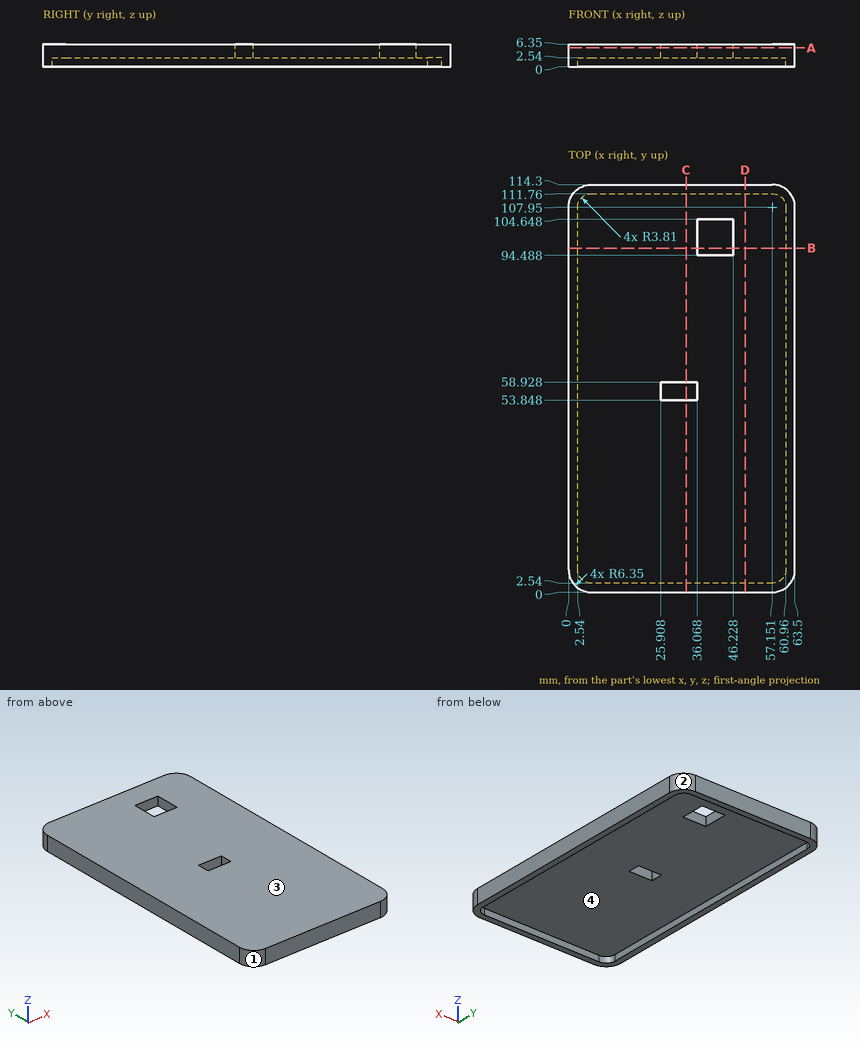
Print and shaded views of the part. All mm, measured from the part's lowest x, y and z. Coordinates: 2 decimals unless noted, no trailing zeros. Write each loop counter-clockwise with the first axis right and the second up, starting at its lowest first coordinate (ties: lowest second). Pieces come first, ordered by that corner, then holes.
(1) Flat gauge pin, fed straight in: pin 1 (4 mm diameter, centred on x = 23.5, y = 80.5, fed in from -Z). Where does the tip first touch, or does it go through?
(2) Cut at A-A, the plane z = 5.25. List the corners of the cut face in (x, y).
(3) Cut at C-C, the plane x = 33. List the corners of the cut face in (y, z).
(4) Cut at D-D, the plane x = 49.5. List the corners of the cut face in (y, z).
(5) Drill centre lines: probe 1 along X at (y, z) = (55.5, 1); probe 2 along Y at (x, z) = (44, 4.5); probe 3 along Y at (x, z) = (27, 5.25). Where is each one in solid material? Low to high.
(6) Two-plate mould, pull along X, no slides. Class the marked faces 1, 2, 3 and 4: +X half, -X half, draft (parallel to the pull), parting line (faces both ways), or undercut.
(7) Cut at B-B, the plane y = 96.5. List the corners of the cut face in (x, z), and give its area (3 significant figures).
Geometry says:
1. pin 1: stops at z = 2.54
2. outline: (0, 6.35) arc R6.35 ccw to (6.35, 0) - (57.15, 0) arc R6.35 ccw to (63.5, 6.35) - (63.5, 107.95) arc R6.35 ccw to (57.15, 114.3) - (6.35, 114.3) arc R6.35 ccw to (0, 107.95) - close; hole (25.91, 53.85) - (36.07, 53.85) - (36.07, 58.93) - (25.91, 58.93) - close; hole (36.07, 94.49) - (46.23, 94.49) - (46.23, 104.65) - (36.07, 104.65) - close
3. outline: (0, 0) - (2.54, 0) - (2.54, 2.54) - (53.85, 2.54) - (53.85, 6.35) - (0, 6.35) - close; (58.93, 2.54) - (111.76, 2.54) - (111.76, 0) - (114.3, 0) - (114.3, 6.35) - (58.93, 6.35) - close
4. outline: (0, 0) - (2.54, 0) - (2.54, 2.54) - (111.76, 2.54) - (111.76, 0) - (114.3, 0) - (114.3, 6.35) - (0, 6.35) - close
5. probe 1: x = 0 to 2.54, 60.96 to 63.5
5. probe 2: y = 0 to 94.49, 104.65 to 114.3
5. probe 3: y = 0 to 53.85, 58.93 to 114.3
6. face 1: -X half
6. face 2: +X half
6. face 3: draft
6. face 4: undercut
7. outline: (0, 0) - (2.54, 0) - (2.54, 2.54) - (36.07, 2.54) - (36.07, 6.35) - (0, 6.35) - close; (46.23, 2.54) - (60.96, 2.54) - (60.96, 0) - (63.5, 0) - (63.5, 6.35) - (46.23, 6.35) - close
7. area: 216 mm2
